```python
from build123d import *

# Parameters (mm, degrees)
EXTRUDE_1_DEPTH     = 7
CUT_EXTRUDE_1_DEPTH = 9
EXTRUDE_5_DEPTH     = 7.2
SKETCH_14_R         = 11.1
CUT_EXTRUDE_2_DEPTH = 235.901017342
SKETCH_15_W         = 30
SKETCH_15_H         = 4
SKETCH_15_W_2       = 35
EXTRUDE_6_DEPTH     = 5
CUT_EXTRUDE_3_DEPTH = 7.2


with BuildPart() as part:
    # Эскиз1 → Бобышка-Вытянуть1 (new body)
    with BuildSketch(Plane(origin=(0, 0, 0), x_dir=(1, 0, 0), z_dir=(0, 1, 0))):
        with BuildLine():
            Line((199.917837119, 0), (30, 0))
            ThreePointArc((30, 0), (-17.429967854, 24.417129656), (-9.746414708, -28.372652332))
            Line((-9.746414708, -28.372652332), (69.918056204, -55.738545445))
            Line((69.918056204, -55.738545445), (199.917837119, -55.499878365))
            ThreePointArc((199.917837119, -55.499878365), (227.75, -27.75), (199.917837119, -0.000121635))
            Line((199.917837119, -0.000121635), (199.917837119, 0))
        make_face()
    extrude(amount=EXTRUDE_1_DEPTH)

    # Эскиз10 → Вырез-Вытянуть1 (cut)
    with BuildSketch(Plane.XZ):
        Polygon((0, 7.3), (-6.321985448, 3.65), (-6.321985448, -3.65), (0, -7.3), (6.321985448, -3.65), (6.321985448, 3.65), align=None)
    extrude(amount=-CUT_EXTRUDE_1_DEPTH, mode=Mode.SUBTRACT)

    # Эскиз11 → Бобышка-Вытянуть5 (add)
    with BuildSketch(Plane(origin=(0, 7, 0), x_dir=(1, 0, 0), z_dir=(0, 1, 0))):
        with BuildLine():
            ThreePointArc((191.546705266, -55.515246957), (170.918554023, -27.776478596), (191.495899106, 0))
            Line((191.495899106, 0), (69.918541879, 0))
            Line((69.918541879, 0), (69.918541879, -55.738544553))
            Line((69.918541879, -55.738544553), (191.546705266, -55.515246957))
        make_face()
    extrude(amount=EXTRUDE_5_DEPTH)

    # Эскиз14 → Вырез-Вытянуть2 (cut, through all)
    with BuildSketch(Plane.XZ):
        with Locations(Location((200, 27.75, 0), (0, 0, 270))):
            Circle(SKETCH_14_R)
    extrude(amount=-CUT_EXTRUDE_2_DEPTH, mode=Mode.SUBTRACT)

    # Эскиз15 → Бобышка-Вытянуть6 (add)
    with BuildSketch(Plane(origin=(0, 14.2, 0), x_dir=(1, 0, 0), z_dir=(0, 1, 0))):
        with Locations((105, -6)):
            Rectangle(SKETCH_15_W, SKETCH_15_H)
        with Locations((150, -6)):
            Rectangle(SKETCH_15_W, SKETCH_15_H)
        with Locations((142.42, -49.573303801)):
            Rectangle(SKETCH_15_W_2, SKETCH_15_H)
    extrude(amount=EXTRUDE_6_DEPTH)

    # Эскиз16 → Вырез-Вытянуть3 (cut)
    with BuildSketch(Plane(origin=(0, 14.2, 0), x_dir=(1, 0, 0), z_dir=(0, 1, 0))):
        Polygon((78.100396808, 0), (69.918541879, 0), (69.918541879, -55.738544553), (120.375042432, -55.645911276), align=None)
    extrude(amount=-CUT_EXTRUDE_3_DEPTH, mode=Mode.SUBTRACT)


solid = part.part
```
Geometry: final body of the model. Coordinates: model frame, mm. A direction names the side the tool comes from. Give positions to 0.01 mm unless a question says otherwise; leave off trailing zeros. Loops run counter-clockwise (first coordinate to the right, second up) from the corner with the lowest first, then second, coordinate; pieces in that order, holes last. Notation, with made-up numbers: (81.5, -13) -> (101.5, -13) arc R10 cw to (101.5, -9) -> close; hole circle Ø4 at (35.25, 80.5). An arc over 180 degrees is marked (long way). Use one line per item in the form item = value.
Item 1: Section query C-C on x = 203. Output: boundary loops of the cut face in (y, z).
A:
outline = (0, 0.16) -> (7, 0.16) -> (7, 17.06) -> (0, 17.06) -> close; (0, 38.44) -> (7, 38.44) -> (7, 55.34) -> (0, 55.34) -> close
Item 2: Access query for faces 5 (the face through (105, 17, 4)), 6 (the face through (116, 7, 0)), 7 (the face through (-3.12, 3.45, 5.5)), 8 (the face through (99.53, 10.65, 28.21)), 9 (the face through (170.924, 10.55, 28.295)). Directions: +Z, -Z, +X, -X, +Y, -Y. A direction counts if a zero-diameter tool reaches every point of the face in a straight line with its end or side. Return the directions, or none.
A:
face_5 = -Z, +X, -X, +Y
face_6 = -Z, +X, +Y, -Y
face_7 = +Y, -Y
face_8 = +Z, -X, +Y
face_9 = +X, +Y
Item 3: Section query D-D on x = 111. Output: boundary loops of the cut face in (y, z), and give its area (3 significant figures).
A:
outline = (0, 0) -> (14.2, 0) -> (14.2, 4) -> (19.2, 4) -> (19.2, 8) -> (14.2, 8) -> (14.2, 43.31) -> (7, 43.31) -> (7, 55.66) -> (0, 55.66) -> close
area = 721 mm^2
Item 4: Section query A-A on y = 16.5. Output: boundary loops of the cut face in (x, z).
A:
outline = (90, 4) -> (120, 4) -> (120, 8) -> (90, 8) -> close; (124.92, 47.57) -> (159.92, 47.57) -> (159.92, 51.57) -> (124.92, 51.57) -> close; (135, 4) -> (165, 4) -> (165, 8) -> (135, 8) -> close
Item 5: Pin query (flat end, axial travel): P1, Ø3, axis at y = 16, z = 6, coming from the -X side; P2, Ø4, axis at x = 155, y = 16, coming from the -Z side; P3, Ø5, axis at x = 134, z = 5.5, coming from the +Y side; P4, Ø2, axis at y = 15.5, z = 6, coming from the +X side. Return the tip coordinate at first contact, or that it passes through.
A:
P1 = 90
P2 = 0
P3 = 19.2
P4 = 165
Item 6: Draft query along Z for faces 1 (the face through (29.528, 3.451, 41.864)), 2 (the face through (-16.67, 3.45, -24.94)), 3 (the face through (44, 7, 12)), 4 (the face through (-3.205, 3.451, -5.449)). Return one class per face: pulls with the +Z half, pulls with the -Z half, needs draft (parallel to the pull), parting line crosses it, or undercut.
A:
face_1 = pulls with the +Z half
face_2 = parting line crosses it
face_3 = needs draft
face_4 = undercut
Item 7: Section query B-B on z = 25. Output: boundary loops of the cut face in (x, y), and give its area (3 significant figures).
A:
outline = (-16.58, 0) -> (189.25, 0) -> (189.25, 7) -> (171.05, 7) -> (171.05, 14.2) -> (97.09, 14.2) -> (97.09, 7) -> (-16.58, 7) -> close; (210.75, 0) -> (227.61, 0) -> (227.61, 7) -> (210.75, 7) -> close
area = 2,090 mm^2
Item 8: Line query: probe 1 along Y at (x, z) = (144, 31.5); probe 2 along Y at (x, z) = (20, 1); probe 3 along Z at (x, y) = (113, 2). Output: solid intervals per line, ascending.
A:
probe_1 = 0 to 14.2
probe_2 = 0 to 7
probe_3 = 0 to 55.66
